```python
from build123d import *

# Parameters (mm, degrees)
SKETCH1_W           = 60.96
SKETCH1_H           = 20.32
SKETCH1_R           = 1
SKETCH1_R_2         = 0.5
BOSS_EXTRUDE1_DEPTH = 1.5
SKETCH1_3_R         = 0.5
CUT_EXTRUDE3_DEPTH  = 0.03


with BuildPart() as part:
    # Sketch1 → Boss-Extrude1 (new body)
    with BuildSketch(Plane(origin=(0, 0, 0), x_dir=(1, 0, 0), z_dir=(0, 1, 0))):
        with Locations((30.48, 10.16)):
            Rectangle(SKETCH1_W, SKETCH1_H)
        with Locations(Location((2.54, 2.54, 0), (0, 0, 270))):  # turned: the seam where the file's is
            Circle(SKETCH1_R, mode=Mode.SUBTRACT)
        with Locations(Location((58.42, 2.54, 0), (0, 0, 270))):  # turned: the seam where the file's is
            Circle(SKETCH1_R, mode=Mode.SUBTRACT)
        with Locations(Location((58.42, 17.78, 0), (0, 0, 270))):  # turned: the seam where the file's is
            Circle(SKETCH1_R, mode=Mode.SUBTRACT)
        with Locations(Location((2.54, 17.78, 0), (0, 0, 270))):  # turned: the seam where the file's is
            Circle(SKETCH1_R, mode=Mode.SUBTRACT)
        with Locations(Location((10.16, 2.54, 0), (0, 0, 270))):  # turned: the seam where the file's is
            Circle(SKETCH1_R_2, mode=Mode.SUBTRACT)
        with Locations(Location((10.16, 17.78, 0), (0, 0, 270))):  # turned: the seam where the file's is
            Circle(SKETCH1_R_2, mode=Mode.SUBTRACT)
    extrude(amount=BOSS_EXTRUDE1_DEPTH)

    # Sketch1_3 → Cut-Extrude3 (cut)
    with BuildSketch(Plane(origin=(0, 0, 0), x_dir=(1, 0, 0), z_dir=(0, 1, 0))):
        with Locations(Location((53.34, 8.57, 0), (0, 0, 270))):  # turned: the seam where the file's is
            Circle(SKETCH1_3_R)
        with Locations(Location((53.34, 11.11, 0), (0, 0, 90))):  # turned: the seam where the file's is
            Circle(SKETCH1_3_R)
    extrude(amount=CUT_EXTRUDE3_DEPTH, mode=Mode.SUBTRACT)


solid = part.part
```
Geometry check sheet. Reference: the model listing, model coordinates, mm. Round coordinates to 2 decimals unless told otherwise and drop trailing zeros. Write each loop counter-clockwise with the first axis right and the second up, starting at its lowest first coordinate (ties: lowest second). Pieces come first, ordered by that corner, then holes. Notation, with made-up numbers: (-30.75, -21.75) -> (1.25, -21.75) arc R22 ccw to (1.25, 3.25) -> close; hole circle Ø6 at (5.5, 61). An arc over 180 degrees is marked (long way). Put each result on its own line as item: value.
1) Thickness scan on probe 1 along X at (y, z) = (1.05, -2.54); probe 2 along X at (y, z) = (0.55, -17); probe 3 along X at (y, z) = (1.25, -3.25). Record the ranges inside material, lowest first. Write a range as from..to.
Recorded:
probe 1: x = 0..1.54, 3.54..9.66, 10.66..57.42, 59.42..60.96
probe 2: x = 0..1.91, 3.17..57.79, 59.05..60.96
probe 3: x = 0..1.84, 3.24..57.72, 59.12..60.96
2) Cross-section at A-A, the plane x = 58.42. Enter the section's corners in (y, z), plus the area to 3 significant figures.
Recorded:
outline: (0, -20.32) -> (1.5, -20.32) -> (1.5, -18.78) -> (0, -18.78) -> close; (0, -16.78) -> (1.5, -16.78) -> (1.5, -3.54) -> (0, -3.54) -> close; (0, -1.54) -> (1.5, -1.54) -> (1.5, 0) -> (0, 0) -> close
area: 24.5 mm2
3) Release check for a two-part mould opening along Z. For faces 1 (the face through (30, 1, 0)), 2 (the face through (57.444, 0.74, -2.757)), 3 (the face through (30, 0, -10)), 4 (the face through (30, 1, -20.32)) record: pulls with the +Z half, pulls with the -Z half, needs draft (parallel to the pull), parting line crosses it, or undercut.
Recorded:
face 1: pulls with the +Z half
face 2: undercut
face 3: needs draft
face 4: pulls with the -Z half
